Could you check a few things on this model? Use its own coordinates, in mm. Face numbers are marked on the shaded views. A direction names the side the tool comes from. Give positions to 0.01 mm unless a question says otherwise; leave off trailing zeros. Loops run counter-clockwise (first coordinate to the right, second up) from the corner with the lowest first, then second, coordinate; pieces in that order, holes last.
1. I need wall thicknesses on line 1 along Z through (x, y) = (1.25, 0); line 2 along X through (y, z) = (-2.5, 4); line 3 along X through (y, z) = (3, 2.5). Which ranges of each line are inside material? Lowest first, please.
2. For P1, Ø2, axis at x = 2, z = 17, coming from the -Y side; P2, Ø1.5, axis at y = -1.5, z = 19.5, coming from the +X side; P3, Ø4, axis at x = 0.5, y = 1, coming from the -Z side; P4, Ø1.5, axis at y = 2.5, z = 29, coming from the -X side, each with a flat end and sliding along its axis, tell me the tip position at first contact or that it passes through.
3. For the marked faces 1 and 2, which set-ups out of +Z, -Z, +X, -X, +Y, -Y let a thin tool reach every point of the face, with its end or its side?
4. Imagine slicing it at C-C (z = 25.5). List the corners of the cut face in (x, y) for me, plus the area to 3 significant figures.
5. Imagine slicing it at A-A (y = 0). List the corners of the cut face in (x, z) for me, plus the area to 3 significant figures.
6. Imagine slicing it at D-D (y = -1.5). List the corners of the cut face in (x, z) for me.
7. Imagine slicing it at B-B (x = 0). List the corners of the cut face in (y, z) for me.
```python
from build123d import *

# Parameters (mm, degrees)
ESQUISSE1_R             = 3.65
BOSS_EXTRU_1_DEPTH      = 35
ENL_V_MAT_EXTRU_1_DEPTH = 4.8


with BuildPart() as part:
    # Esquisse1 → Boss.-Extru.1 (new body)
    with BuildSketch(Plane.XY):
        Circle(ESQUISSE1_R)
    extrude(amount=BOSS_EXTRU_1_DEPTH)

    # Esquisse2 → Enlèv. mat.-Extru.1 (cut)
    with BuildSketch(Plane(origin=(0, 0, 0), x_dir=(-1, 0, 0), z_dir=(0, 0, -1))):
        with BuildLine():
            Line((1.75, 4), (1.75, -4))
            ThreePointArc((1.75, -4), (0, -5.75), (-1.75, -4))
            Line((-1.75, -4), (-1.75, 4))
            ThreePointArc((-1.75, 4), (0, 5.75), (1.75, 4))
        make_face()
    extrude(amount=-ENL_V_MAT_EXTRU_1_DEPTH, mode=Mode.SUBTRACT)


solid = part.part
```
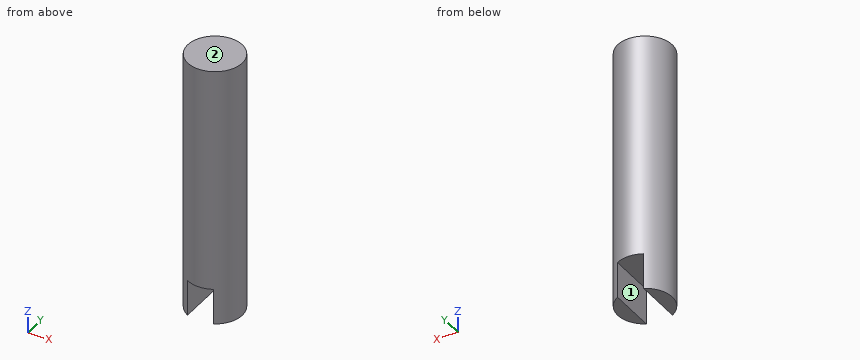
Derived:
1. line 1: z = 4.8 to 35
1. line 2: x = -2.66 to -1.75, 1.75 to 2.66
1. line 3: x = -2.08 to -1.75, 1.75 to 2.08
2. P1: stops at y = -3.51
2. P2: stops at x = 3.57
2. P3: stops at z = 0
2. P4: stops at x = -3.2
3. face 1: -Z, +Y, -Y
3. face 2: +Z, +X, -X, +Y, -Y
4. outline: circle Ø7.3 at (0, 0)
4. area: 41.9 mm2
5. outline: (-3.65, 0) - (-1.75, 0) - (-1.75, 4.8) - (1.75, 4.8) - (1.75, 0) - (3.65, 0) - (3.65, 35) - (-3.65, 35) - close
5. area: 239 mm2
6. outline: (-3.33, 0) - (-1.75, 0) - (-1.75, 4.8) - (1.75, 4.8) - (1.75, 0) - (3.33, 0) - (3.33, 35) - (-3.33, 35) - close
7. outline: (-3.65, 4.8) - (3.65, 4.8) - (3.65, 35) - (-3.65, 35) - close
